```python
from build123d import *

# Parameters (mm, degrees)
SKETCH1_W               = 93
SKETCH1_H               = 62.25
BOSS_EXTRUDE1_DEPTH     = 4
CUT_EXTRUDE1_DEPTH      = 1.75
CUT_EXTRUDE2_DEPTH      = 112.933574052
SKETCH7_R               = 1.15
CUT_EXTRUDE3_DEPTH      = 112.982420495
SKETCH8_W               = 93
SKETCH8_H               = 62.25
SKETCH8_W_2             = 87
SKETCH8_H_2             = 56.25
BOSS_EXTRUDE3_DEPTH     = 10
BOSS_EXTRUDE7_START     = -14
SKETCH16_W              = 6.5
SKETCH16_H              = 4.5
SKETCH16_H_2            = 2
SKETCH16_W_2            = 4.5
BOSS_EXTRUDE7_DEPTH     = 14
SKETCH9_W               = 16
SKETCH9_H               = 7.25
SKETCH9_W_2             = 13.5
SKETCH9_H_2             = 9
CUT_EXTRUDE4_DEPTH      = 3
CUT_EXTRUDE5_DEPTH      = 1.5
CUT_EXTRUDE6_DEPTH      = 113.356853374
CUT_EXTRUDE6_DEPTH_BACK = 5
BOSS_EXTRUDE4_DEPTH     = 1
BOSS_EXTRUDE5_DEPTH     = 4
SKETCH14_W              = 5
SKETCH14_H              = 3
CUT_EXTRUDE8_DEPTH      = 8.5
BOSS_EXTRUDE6_DEPTH     = 0.5
SKETCH17_W              = 6.5
SKETCH17_H              = 4.5
CUT_EXTRUDE9_DEPTH      = 1.75
SKETCH18_R              = 1.75
BOSS_EXTRUDE8_DEPTH     = 6.4
SKETCH19_R              = 1.25
CUT_EXTRUDE10_DEPTH     = 4


with BuildPart() as part:
    # Sketch1 → Boss-Extrude1 (new body)
    with BuildSketch(Plane(origin=(0, 0, 0), x_dir=(1, 0, 0), z_dir=(0, 1, 0))):
        with Locations((46.5, 31.125)):
            Rectangle(SKETCH1_W, SKETCH1_H)
        Polygon((7, 5), (88, 5), (88, 57.25), (40.5, 57.25), (40.5, 26.5), (7, 26.5), align=None, mode=Mode.SUBTRACT)
    extrude(amount=BOSS_EXTRUDE1_DEPTH)

    # Sketch5 → Cut-Extrude1 (cut)
    with BuildSketch(Plane(origin=(0, 4, 0), x_dir=(1, 0, 0), z_dir=(0, 1, 0))):
        Polygon((40.5, 26.5), (15, 26.5), (15, 36.5), (5, 36.5), (5, 57.25), (30.5, 57.25), (30.5, 49.25), (38.5, 49.25), (38.5, 57.25), (40.5, 57.25), align=None)
    extrude(amount=-CUT_EXTRUDE1_DEPTH, mode=Mode.SUBTRACT)

    # Sketch6 → Cut-Extrude2 (cut, through all)
    with BuildSketch(Plane(origin=(0, 2.25, 0), x_dir=(1, 0, 0), z_dir=(0, 1, 0))):
        Polygon((30.5, 49.25), (30, 49.25), (30, 38.5), (20, 38.5), (20, 29.5), (28.25, 29.5), (36.5, 29.5), (36.5, 39.375), (36.5, 49.25), align=None)
    extrude(amount=-CUT_EXTRUDE2_DEPTH, mode=Mode.SUBTRACT)

    # Sketch7 → Cut-Extrude3 (cut, through all)
    with BuildSketch(Plane(origin=(0, 4, 0), x_dir=(1, 0, 0), z_dir=(0, 1, 0))):
        with Locations(Location((8.25, 33, 0), (0, 0, 270))):
            Circle(SKETCH7_R)
        with Locations(Location((34.75, 51.5, 0), (0, 0, 270))):
            Circle(SKETCH7_R)
    extrude(amount=-CUT_EXTRUDE3_DEPTH, mode=Mode.SUBTRACT)

    # Sketch8 → Boss-Extrude3 (add)
    with BuildSketch(Plane.XZ):
        with Locations((46.5, -31.125)):
            Rectangle(SKETCH8_W, SKETCH8_H)
        with Locations((46.5, -31.125)):
            Rectangle(SKETCH8_W_2, SKETCH8_H_2, mode=Mode.SUBTRACT)
    extrude(amount=BOSS_EXTRUDE3_DEPTH)

    # Sketch16 → Boss-Extrude7 (add)
    with BuildSketch(Plane(origin=(0, 4, 0), x_dir=(1, 0, 0), z_dir=(0, 1, 0)).offset(BOSS_EXTRUDE7_START)):
        with Locations((66.5, 7.25)):
            Rectangle(SKETCH16_W, SKETCH16_H)
        with Locations((66.5, 4)):
            Rectangle(SKETCH16_W, SKETCH16_H_2)
        with Locations((66.5, 55)):
            Rectangle(SKETCH16_W, SKETCH16_H)
        with Locations((66.5, 58.25)):
            Rectangle(SKETCH16_W, SKETCH16_H_2)
        with Locations((8.25, 58.25)):
            Rectangle(SKETCH16_W, SKETCH16_H_2)
        Polygon((5, 57.25), (5, 52.75), (7, 52.75), (11.5, 52.75), (11.5, 57.25), align=None)
        with Locations((9.25, 7.25)):
            Rectangle(SKETCH16_W_2, SKETCH16_H)
        Polygon((7, 5), (7, 9.5), (5, 9.5), (5, 3), (11.5, 3), (11.5, 5), align=None)
    extrude(amount=BOSS_EXTRUDE7_DEPTH)

    # Sketch9 → Cut-Extrude4 (cut)
    with BuildSketch(Plane(origin=(93, 0, 0), x_dir=(0, 0, -1), z_dir=(1, 0, 0))):
        with Locations((13.25, -6.375)):
            Rectangle(SKETCH9_W, SKETCH9_H)
        with Locations((32, -5.5)):
            Rectangle(SKETCH9_W_2, SKETCH9_H_2)
        with Locations((49.75, -5.5)):
            Rectangle(SKETCH9_W_2, SKETCH9_H_2)
    extrude(amount=-CUT_EXTRUDE4_DEPTH, mode=Mode.SUBTRACT)

    # Sketch10 → Cut-Extrude5 (cut)
    with BuildSketch(Plane(origin=(93, 0, 0), x_dir=(0, 0, -1), z_dir=(1, 0, 0))):
        Polygon((25.25, -10), (25.25, -1), (38.75, -1), (38.75, -10), (40.25, -10), (40.25, 0.5), (23.75, 0.5), (23.75, -10), align=None)
        Polygon((43, -10), (43, -1), (56.5, -1), (56.5, -10), (58, -10), (58, 0.5), (41.5, 0.5), (41.5, -10), align=None)
    extrude(amount=-CUT_EXTRUDE5_DEPTH, mode=Mode.SUBTRACT)

    # Sketch11 → Cut-Extrude6 (cut, two sides: drawn at the far end of the back side and taken through both)
    with BuildSketch(Plane(origin=(93, 0, 0), x_dir=(0, 0, -1), z_dir=(1, 0, 0)).offset(-CUT_EXTRUDE6_DEPTH_BACK)):
        with BuildLine():
            Line((29.5, 85.233770081), (29.5, 4))
            ThreePointArc((29.5, 4), (31.125, 2.375), (32.75, 4))
            Line((32.75, 4), (32.75, 85.233770081))
            Line((32.75, 85.233770081), (32.75, 247.701310244))
            Line((32.75, 247.701310244), (29.5, 247.701310244))
            Line((29.5, 247.701310244), (29.5, 85.233770081))
        make_face()
    extrude(amount=CUT_EXTRUDE6_DEPTH + CUT_EXTRUDE6_DEPTH_BACK, mode=Mode.SUBTRACT)

    # Sketch12 → Boss-Extrude4 (add)
    with BuildSketch(Plane(origin=(0, -10, 0), x_dir=(-1, 0, 0), z_dir=(0, -1, 0))):
        Polygon((-20, 62.25), (-14, 62.25), (-14, 61.25), (-13, 61.25), (-13, 60.25), (-14, 60.25), (-14, 59.25), (-20, 59.25), (-20, 60.25), (-21, 60.25), (-21, 61.25), (-20, 61.25), align=None)
    extrude(amount=BOSS_EXTRUDE4_DEPTH)

    # Sketch13 → Boss-Extrude5 (add)
    with BuildSketch(Plane.XZ.offset(10)):
        Polygon((20, -3), (11, -3), (11, -2), (10, -2), (10, -1), (11, -1), (11, 0), (20, 0), (20, -1), (21, -1), (21, -2), (20, -2), align=None)
    extrude(amount=BOSS_EXTRUDE5_DEPTH)

    # Sketch14 → Cut-Extrude8 (cut)
    with BuildSketch(Plane.ZY):
        with Locations((-41, 2.5)):
            Rectangle(SKETCH14_W, SKETCH14_H)
    extrude(amount=-CUT_EXTRUDE8_DEPTH, mode=Mode.SUBTRACT)

    # Sketch15 → Boss-Extrude6 (add)
    with BuildSketch(Plane.XZ.offset(10)):
        Polygon((62.5, -3), (55, -3), (55, -2), (54, -2), (54, -1), (55, -1), (55, 0), (62.5, 0), (62.5, -1), (63.5, -1), (63.5, -2), (62.5, -2), align=None)
    extrude(amount=BOSS_EXTRUDE6_DEPTH)

    # Sketch17 → Cut-Extrude9 (cut)
    with BuildSketch(Plane(origin=(0, 4, 0), x_dir=(1, 0, 0), z_dir=(0, 1, 0))):
        with Locations((8.25, 55)):
            Rectangle(SKETCH17_W, SKETCH17_H)
    extrude(amount=-CUT_EXTRUDE9_DEPTH, mode=Mode.SUBTRACT)

    # Sketch18 → Boss-Extrude8 (add)
    with BuildSketch(Plane(origin=(0, -10, 0), x_dir=(-1, 0, 0), z_dir=(0, -1, 0))):
        with Locations(Location((-8.5, 55.75, 0), (0, 0, 90))):
            Circle(SKETCH18_R)
        with Locations(Location((-66.5, 55.75, 0), (0, 0, 90))):
            Circle(SKETCH18_R)
        with Locations(Location((-66.5, 6.5, 0), (0, 0, 270))):
            Circle(SKETCH18_R)
        with Locations(Location((-8.5, 6.5, 0), (0, 0, 270))):
            Circle(SKETCH18_R)
    extrude(amount=BOSS_EXTRUDE8_DEPTH)

    # Sketch19 → Cut-Extrude10 (cut)
    with BuildSketch(Plane.XZ.offset(16.4)):
        with Locations(Location((8.5, -6.5, 0), (0, 0, 270))):
            Circle(SKETCH19_R)
        with Locations(Location((8.5, -55.75, 0), (0, 0, 270))):
            Circle(SKETCH19_R)
        with Locations(Location((66.5, -55.75, 0), (0, 0, 270))):
            Circle(SKETCH19_R)
        with Locations(Location((66.5, -6.5, 0), (0, 0, 270))):
            Circle(SKETCH19_R)
    extrude(amount=-CUT_EXTRUDE10_DEPTH, mode=Mode.SUBTRACT)


solid = part.part
```
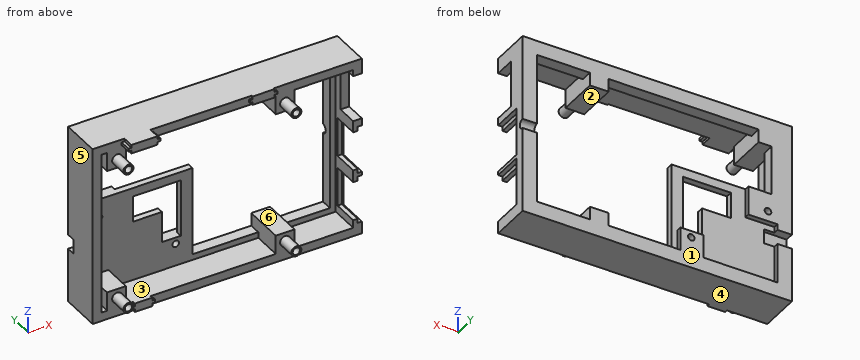
CAD build for the part. Positions are in the model's coordinates, mm. Face numbers are marked on the shaded views. A direction names the side the tool comes from. Coordinates: 2 decimals unless noted, no trailing zeros. Order: outer loops, then holes, each group sorted by start corner. A loop starts at its lowest first (then second) coordinate and runs counter-clockwise, first axis right, second up. Notation, with made-up numbers: (-2.75, -0.5) -> (51.25, -0.5) arc R29 cw to (51.25, 26.5) -> close; hole circle Ø7 at (55, 54). An arc over 180 degrees is marked (long way). Use one line per item in the form item = value. Start each with the question number.
1) Pull direction X, two halves, no side cores. Call the marked faces 4, 5 and 6: +X half, -X half, draft (parallel to the pull), parting line (faces both ways), or undercut.
2) Band-saw the part on C-C on x = 60. Give the cut face in (y, z), then the cut area to 4 significant figures.
3) Drill centre lines: L1, parallel to Z at x = 66.5, y = -14.95; L2, parallel to X at y = -13.4, z = -55.75; L3, parallel to Z at x = 48.5, y = 3.25. Where is each one in solid material? Low to high. Write a range as [from, to].
4) Band-saw the part on D-D on z = -28.5. Give the cut face in (x, y), then the cut area to 3 significant figures.
5) Drop flat-ended pins along their axis: pin 1 (1.5 mm diameter, centred on x = 91.5, z = -22.5, fed in from -Y); pin 2 (2 mm diameter, centred on y = -11.5, z = -27, fed in from -X); pin 3 (0.8 mm diameter, centred on y = -10.5, z = -60.5, fed in from -X); pin 4 (0.8 mm diameter, centred on y = -11, z = -2.5, fed in from +X). Give the stop position or say it passes through.
6) Band-saw the part on A-A on x = 34.75. Give the cut face in (y, z).
7) Tool access for the marked faces 1, 2 and 3: list every direction of +Z, -Z, +X, -X, +Y, -Y with a clear straight run to the whole face (end or side of a thin tool).
8) Band-saw the part on B-B on z = -51.5. Give the cut face in (x, y).
Entries:
q1.face_4 = draft
q1.face_5 = -X half
q1.face_6 = undercut
q2.outline = (-10.5, -3) -> (0, -3) -> (0, -5) -> (4, -5) -> (4, 0) -> (-10.5, 0) -> close; (-10, -62.25) -> (4, -62.25) -> (4, -57.25) -> (0, -57.25) -> (0, -59.25) -> (-10, -59.25) -> close
q2.area = 101.5 mm2
q3.L1 = [-57.5, -57], [-54.5, -54], [-8.25, -7.75], [-5.25, -4.75]
q3.L2 = [6.75, 7.25], [9.75, 10.25], [64.75, 65.25], [67.75, 68.25]
q3.L3 = [-62.25, -57.25], [-5, 0]
q4.outline = (0, -10) -> (3, -10) -> (3, 0) -> (40.5, 0) -> (40.5, 2.25) -> (15, 2.25) -> (15, 4) -> (0, 4) -> close; (88, 0) -> (90, 0) -> (90, -1) -> (91.5, -1) -> (91.5, 0.5) -> (93, 0.5) -> (93, 4) -> (88, 4) -> close
q4.area = 168 mm2
q5.pin_1 = -10
q5.pin_2 = through
q5.pin_3 = 13
q5.pin_4 = 20
q6.outline = (-10, -62.25) -> (4, -62.25) -> (4, -52.65) -> (0, -52.65) -> (0, -59.25) -> (-10, -59.25) -> close; (-10, -3) -> (0, -3) -> (0, -5) -> (4, -5) -> (4, 0) -> (-10, 0) -> close; (0, -50.35) -> (4, -50.35) -> (4, -49.25) -> (0, -49.25) -> close; (0, -29.5) -> (2.25, -29.5) -> (2.25, -26.5) -> (0, -26.5) -> close
q7.face_1 = +Z, -Z, +X, -X, +Y
q7.face_2 = +Y, -Y
q7.face_3 = -Y
q8.outline = (0, -10) -> (3, -10) -> (3, 0) -> (33.6, 0) -> (33.6, 4) -> (30.5, 4) -> (30.5, 2.25) -> (5, 2.25) -> (5, 4) -> (0, 4) -> close; (35.9, 0) -> (40.5, 0) -> (40.5, 2.25) -> (38.5, 2.25) -> (38.5, 4) -> (35.9, 4) -> close; (88, 0) -> (90, 0) -> (90, -1) -> (91.5, -1) -> (91.5, 0.5) -> (93, 0.5) -> (93, 4) -> (88, 4) -> close
